Can you work these out from the model? Positions are in its coordinate system, mm. Coordinates: 2 decimals unless noted, no trailing zeros. Write each loop counter-clockwise with the first axis right and the second up, starting at its lowest first coordinate (ties: lowest second). Pieces come first, ordered by that corner, then holes. Notation, with made-up numbers: (-17.5, 56) - (-12.5, 56) arc R13 cw to (-12.5, 72) - close; hole circle Ø4 at (-36.5, -22.75). An arc over 180 degrees is marked (long way). Use one line per item in the form item = value. Start each with the question number.
(1) If I drill on probe 1 along X at (y, z) = (-41.5, 1.5); probe 2 along Y at (x, z) = (0, 0.5); probe 3 along X at (y, z) = (-10, 1.2), over which ranges is the centre line in solid material (lowest first)? Write a range as from..to.
(2) If we section it at B-B on x = 0: Please give me the cut outline in (y, z).
(3) If we section it at A-A on z = 2.2: Please give me the cut outline in (x, y).
```python
from build123d import *

# Parameters (mm, degrees)
F0_R         = 51
F1_DEPTH     = 3
F2_T1_DEPTH  = 82.316462509
F2_T3_DEPTH  = 82.316462509
F2_T6_ANGLE  = 90
F2_T8_ANGLE  = 90
F2_T10_ANGLE = 90
F2_T12_ANGLE = 90


# Not quite as in the source:
# - a fillet or chamfer that OpenCascade refuses, or shapes differently, is made with other operations: its cross-section is extruded or revolved along the edge and cut away or added


with BuildPart() as f1:
    # F0 (on Top) → F1 (new body)
    with BuildSketch(Plane.XY):
        with BuildLine():
            Line((41.1582312545, 53.5), (-41.1582312545, 53.5))
            ThreePointArc((-41.1582312545, 53.5), (-49.8851796263, 49.8851796263), (-53.5, 41.1582312545))
            Line((-53.5, 41.1582312545), (-53.5, -41.1582312545))
            ThreePointArc((-53.5, -41.1582312545), (-49.8851796263, -49.8851796263), (-41.1582312545, -53.5))
            Line((-41.1582312545, -53.5), (41.1582312545, -53.5))
            ThreePointArc((41.1582312545, -53.5), (49.8851796263, -49.8851796263), (53.5, -41.1582312545))
            Line((53.5, -41.1582312545), (53.5, 41.1582312545))
            ThreePointArc((53.5, 41.1582312545), (49.8851796263, 49.8851796263), (41.1582312545, 53.5))
        make_face()
        with BuildLine():
            ThreePointArc((-40.3050865276, -43.8406204336), (-43.8406204336, -43.8406204336), (-43.8406204336, -40.3050865276))
            Line((-43.8406204336, -40.3050865276), (-42.4264068712, -38.8908729653))
            ThreePointArc((-42.4264068712, -38.8908729653), (-38.8908729653, -38.8908729653), (-38.8908729653, -42.4264068712))
            Line((-38.8908729653, -42.4264068712), (-40.3050865276, -43.8406204336))
        make_face(mode=Mode.SUBTRACT)
        Circle(F0_R, mode=Mode.SUBTRACT)
        with BuildLine():
            ThreePointArc((43.8406204336, -40.3050865276), (43.8406204336, -43.8406204336), (40.3050865276, -43.8406204336))
            Line((40.3050865276, -43.8406204336), (38.8908729653, -42.4264068712))
            ThreePointArc((38.8908729653, -42.4264068712), (38.8908729653, -38.8908729653), (42.4264068712, -38.8908729653))
            Line((42.4264068712, -38.8908729653), (43.8406204336, -40.3050865276))
        make_face(mode=Mode.SUBTRACT)
        with BuildLine():
            ThreePointArc((-43.8406204336, 40.3050865276), (-43.8406204336, 43.8406204336), (-40.3050865276, 43.8406204336))
            Line((-40.3050865276, 43.8406204336), (-38.8908729653, 42.4264068712))
            ThreePointArc((-38.8908729653, 42.4264068712), (-38.8908729653, 38.8908729653), (-42.4264068712, 38.8908729653))
            Line((-42.4264068712, 38.8908729653), (-43.8406204336, 40.3050865276))
        make_face(mode=Mode.SUBTRACT)
        with BuildLine():
            ThreePointArc((40.3050865276, 43.8406204336), (43.8406204336, 43.8406204336), (43.8406204336, 40.3050865276))
            Line((43.8406204336, 40.3050865276), (42.4264068712, 38.8908729653))
            ThreePointArc((42.4264068712, 38.8908729653), (38.8908729653, 38.8908729653), (38.8908729653, 42.4264068712))
            Line((38.8908729653, 42.4264068712), (40.3050865276, 43.8406204336))
        make_face(mode=Mode.SUBTRACT)
    extrude(amount=F1_DEPTH)

    # F2: fillet of radius 1.5 on 8 edges, made by hand

    # F2_s2 → F2_t1 (cut)
    with BuildSketch(Plane.XZ.offset(-41.1582312545)):
        with BuildLine():
            ThreePointArc((-53.5, 1.5), (-53.0606601718, 2.5606601718), (-52, 3))
            Line((-52, 3), (-53.5, 3))
            Line((-53.5, 3), (-53.5, 1.5))
        make_face()
        with BuildLine():
            ThreePointArc((53.5, 1.5), (53.0606601718, 2.5606601718), (52, 3))
            Line((52, 3), (53.5, 3))
            Line((53.5, 3), (53.5, 1.5))
        make_face()
    extrude(amount=F2_T1_DEPTH, mode=Mode.SUBTRACT)

    # F2_s4 → F2_t3 (cut)
    with BuildSketch(Plane.YZ.offset(-41.1582312545)):
        with BuildLine():
            ThreePointArc((53.5, 1.5), (53.0606601718, 2.5606601718), (52, 3))
            Line((52, 3), (53.5, 3))
            Line((53.5, 3), (53.5, 1.5))
        make_face()
        with BuildLine():
            ThreePointArc((-53.5, 1.5), (-53.0606601718, 2.5606601718), (-52, 3))
            Line((-52, 3), (-53.5, 3))
            Line((-53.5, 3), (-53.5, 1.5))
        make_face()
    extrude(amount=F2_T3_DEPTH, mode=Mode.SUBTRACT)

    # F2_s5 → F2_t6 (revolve, cut)
    with BuildSketch(Plane.YZ.offset(-41.1582312545)):
        with BuildLine():
            ThreePointArc((53.5, 1.5), (53.0606601718, 2.5606601718), (52, 3))
            Line((52, 3), (53.5, 3))
            Line((53.5, 3), (53.5, 1.5))
        make_face()
    revolve(axis=Axis((-41.1582312545, 41.1582312545, 3), (0, 0, 1)), revolution_arc=F2_T6_ANGLE, mode=Mode.SUBTRACT)

    # F2_s7 → F2_t8 (revolve, cut)
    with BuildSketch(Plane.XZ.offset(-41.1582312545)):
        with BuildLine():
            ThreePointArc((53.5, 1.5), (53.0606601718, 2.5606601718), (52, 3))
            Line((52, 3), (53.5, 3))
            Line((53.5, 3), (53.5, 1.5))
        make_face()
    revolve(axis=Axis((41.1582312545, 41.1582312545, 3), (0, 0, 1)), revolution_arc=F2_T8_ANGLE, mode=Mode.SUBTRACT)

    # F2_s9 → F2_t10 (revolve, cut)
    with BuildSketch(Plane.XZ.offset(41.1582312545)):
        with BuildLine():
            ThreePointArc((-53.5, 1.5), (-53.0606601718, 2.5606601718), (-52, 3))
            Line((-52, 3), (-53.5, 3))
            Line((-53.5, 3), (-53.5, 1.5))
        make_face()
    revolve(axis=Axis((-41.1582312545, -41.1582312545, 3), (0, 0, 1)), revolution_arc=F2_T10_ANGLE, mode=Mode.SUBTRACT)

    # F2_s11 → F2_t12 (revolve, cut)
    with BuildSketch(Plane.YZ.offset(41.1582312545)):
        with BuildLine():
            ThreePointArc((-53.5, 1.5), (-53.0606601718, 2.5606601718), (-52, 3))
            Line((-52, 3), (-53.5, 3))
            Line((-53.5, 3), (-53.5, 1.5))
        make_face()
    revolve(axis=Axis((41.1582312545, -41.1582312545, 3), (0, 0, 1)), revolution_arc=F2_T12_ANGLE, mode=Mode.SUBTRACT)

    # F2_s13 → F2_t14 (revolve, cut)
    with BuildSketch(Plane.XZ):
        with BuildLine():
            ThreePointArc((51, 1.5), (51.4393398282, 2.5606601718), (52.5, 3))
            Line((52.5, 3), (51, 3))
            Line((51, 3), (51, 1.5))
        make_face()
    revolve(axis=Axis((0, 0, 3), (0, 0, 1)), mode=Mode.SUBTRACT)


solid = f1.part
```
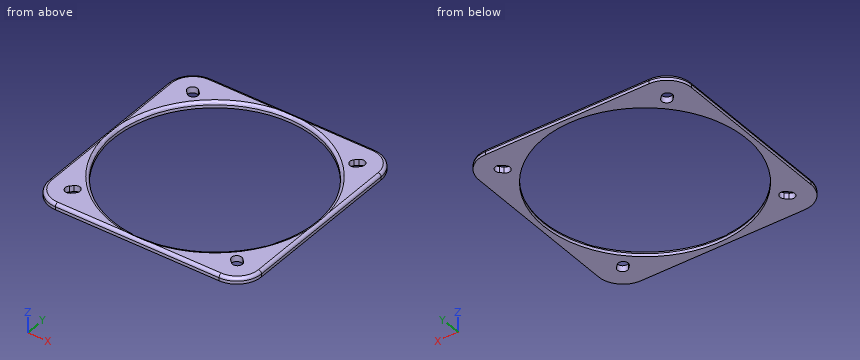
Reported:
q1.probe_1 = -53.5..-44.51, -38.3..-29.64, 29.64..38.3, 44.51..53.5
q1.probe_2 = -53.5..-51, 51..53.5
q1.probe_3 = -53.5..-50.01, 50.01..53.5
q2.outline = (-53.5, 0) - (-51, 0) - (-51, 1.5) arc R1.5 ccw to (-52.25, 2.98) arc R1.5 ccw to (-53.5, 1.5) - close; (51, 0) - (53.5, 0) - (53.5, 1.5) arc R1.5 ccw to (52.25, 2.98) arc R1.5 ccw to (51, 1.5) - close
q3.outline = (-53.33, -41.16) arc R12.17 ccw to (-41.16, -53.33) - (41.16, -53.33) arc R12.17 ccw to (53.33, -41.16) - (53.33, 41.16) arc R12.17 ccw to (41.16, 53.33) - (-41.16, 53.33) arc R12.17 ccw to (-53.33, 41.16) - close; hole circle Ø102.35 at (0, 0); hole (-43.84, -40.31) arc R2.5 ccw to (-40.31, -43.84) - (-38.89, -42.43) arc R2.5 ccw to (-42.43, -38.89) - close; hole (-43.84, 40.31) - (-42.43, 38.89) arc R2.5 ccw to (-38.89, 42.43) - (-40.31, 43.84) arc R2.5 ccw to start; hole (38.89, -42.43) - (40.31, -43.84) arc R2.5 ccw to (43.84, -40.31) - (42.43, -38.89) arc R2.5 ccw to start; hole (38.89, 42.43) arc R2.5 ccw to (42.43, 38.89) - (43.84, 40.31) arc R2.5 ccw to (40.31, 43.84) - close
